Design review of the part built by this model. Coordinates are the model's own, in mm. Face numbers are marked on the shaded views. A direction names the side the tool comes from. Round coordinates to 2 decimals unless told otherwise and drop trailing zeros. Write each loop counter-clockwise with the first axis right and the second up, starting at its lowest first coordinate (ties: lowest second). Pieces come first, ordered by that corner, then holes. Notation, with made-up numbers: M -32.75,75 L 12.25,75 A20 cw 12.25,106 Z; hole C 62.5,-1.5 d2. An arc over 180 degrees is marked long. One line per question, with ' | ' between items. Start each with the question number.
Item 1: Add section A-A, the plane x = -1.25. State the section outline as (y, z) points.
Item 2: Add section D-D, the plane y = 0.9. State the section outline as (x, z) points.
Item 3: Machinability: for the marked faces 4 and 5, which of the approach directions +Z, -Z, +X, -X, +Y, -Y give a long, thin tool a straight path to every point of the face, cutting with its end or side? Answer none if there is none.
Item 4: Add section B-B, the plane z = 0. State the section outline as (x, y) points, and give its area (3 significant figures).
Item 5: Insertion check: pin 1 Ø2 at (y, z) = (1.5, 3) entering from +X; pin 2 Ø9.5 at (x, z) = (2, 2.5) entering from -Y; pin 3 Ø1.8 at (x, z) = (0, -7.5) entering from -Y. Each pin has a flat end and moves straight along its axis. Give the tip position at first contact, or say it passes through.
Item 6: Add section C-C, the plane y = 2.6. State the section outline as (x, z) points, and give its area (3 significant figures).
Item 7: Draft analysis for pull direction Z (two halves, no side actions). For the marked faces 1, 2 and 3, state which applies: released by +Z, released by -Z, zero draft, split by the parting line, or undercut.
Item 8: For L1, parallel to X at y = 1.1, z = 0; L2, parallel to X at y = 2.35, z = 0; L3, parallel to Y at x = -7.25, z = 2, list the stretches that pass through material, from the lowest coordinate up.
```python
from build123d import *

# Parameters (mm, degrees)
ESQUISSE1_R      = 5
EXTRUSION1_DEPTH = 2
ESQUISSE2_R      = 9.5
EXTRUSION2_DEPTH = 1.5
ESQUISSE3_R      = 2.5
ESQUISSE3_R_2    = 1
EXTRUSION3_DEPTH = 14.883443377


with BuildPart() as part:
    # Esquisse1 → Extrusion1 (new body)
    with BuildSketch(Plane(origin=(0, 0, 0), x_dir=(1, 0, 0), z_dir=(0, 1, 0))):
        with Locations(Location((0, 0, 0), (0, 0, 270))):
            Circle(ESQUISSE1_R)
    extrude(amount=EXTRUSION1_DEPTH)

    # Esquisse2 → Extrusion2 (add)
    with BuildSketch(Plane(origin=(0, 2, 0), x_dir=(-1, 0, 0), z_dir=(0, 1, 0))):
        with Locations(Location((0, 0, 0), (0, 0, 90))):
            Circle(ESQUISSE2_R)
    extrude(amount=EXTRUSION2_DEPTH)

    # Esquisse3 → Extrusion3 (cut, through all)
    with BuildSketch(Plane(origin=(0, 3.5, 0), x_dir=(-1, 0, 0), z_dir=(0, 1, 0))):
        with Locations(Location((0, 0, 0), (0, 0, 90))):
            Circle(ESQUISSE3_R)
        with Locations(Location((0, -7.5, 0), (0, 0, 90))):
            Circle(ESQUISSE3_R_2)
        with Locations(Location((0, 7.5, 0), (0, 0, 90))):
            Circle(ESQUISSE3_R_2)
    extrude(amount=-EXTRUSION3_DEPTH, mode=Mode.SUBTRACT)


solid = part.part
```
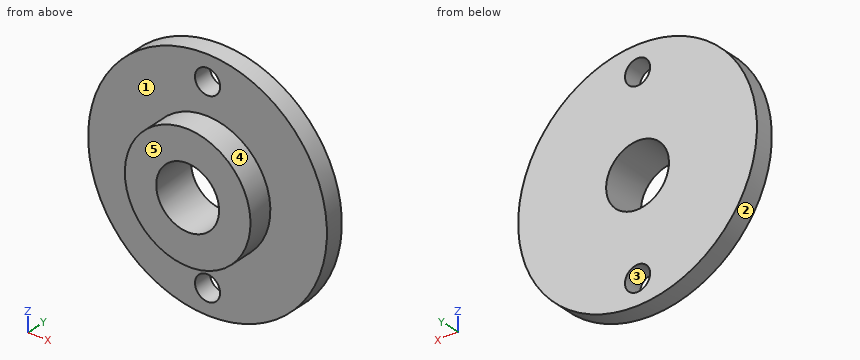
Computed values:
1) outline: M 0,-4.84 L 2,-4.84 L 2,-9.42 L 3.5,-9.42 L 3.5,-2.17 L 0,-2.17 Z; M 0,2.17 L 3.5,2.17 L 3.5,9.42 L 2,9.42 L 2,4.84 L 0,4.84 Z
2) outline: C 0,0 d10; hole C 0,0 d5
3) face 4: -Y | face 5: +Z, -Z, +X, -X, -Y
4) outline: M -9.5,2 L -5,2 L -5,0 L -2.5,0 L -2.5,3.5 L -9.5,3.5 Z; M 2.5,0 L 5,0 L 5,2 L 9.5,2 L 9.5,3.5 L 2.5,3.5 Z | area: 31.0 mm^2
5) pin 1: stops at x = 9.26 | pin 2: stops at y = 0 | pin 3: passes through
6) outline: C 0,0 d19; hole C 0,0 d5; hole C 0,-7.5 d2; hole C 0,7.5 d2 | area: 258 mm^2
7) face 1: zero draft | face 2: split by the parting line | face 3: undercut
8) L1: x = -5 to -2.5, 2.5 to 5 | L2: x = -9.5 to -2.5, 2.5 to 9.5 | L3: y = 2 to 3.5
